Autodesk Inventor part; units mm, degrees
ref_plane "YZ Plane" through (0, 0, 0) normal (1, 0, 0) x (0, 1, 0)
ref_plane "XZ Plane" through (0, 0, 0) normal (0, 1, 0) x (-1, 0, 0)
ref_plane "XY Plane" through (0, 0, 0) normal (0, 0, 1) x (1, 0, 0)
sketch "스케치1" plane through (0, 0, 0) normal (0, 0, 1) x (1, 0, 0)
  line L0 (16.3992, -9.8355) -> (-16.3992, -9.8355)
  line L1 (-16.3992, -9.8355) -> (-16.3992, 9.8355)
  line L2 (-16.3992, 9.8355) -> (16.3992, 9.8355)
  line L3 (16.3992, 9.8355) -> (16.3992, -9.8355)
  line L4 (16.3992, -9.8355) -> (-16.3992, 9.8355) construction
  line L5 (-16.3992, -9.8355) -> (16.3992, 9.8355) construction
  point P0 (0, 0)
extrude "돌출1" add sketch "스케치1" along normal blind 15
sketch "스케치2" plane through (0, 0, 15) normal (0, 0, 1) x (1, 0, 0)
  line L0 (-16.3992, 9.8355) -> (-16.3992, -9.8355)
  line L1 (-16.3992, -9.8355) -> (16.3992, -9.8355)
  line L2 (-16.3992, -0.8122) -> (-1.2307, -0.8122)
  line L3 (-1.2307, -0.8122) -> (-1.2307, -9.8355)
  line L4 (-1.2307, -9.8355) -> (-16.3992, -9.8355)
  line L5 (-16.3992, -9.8355) -> (-16.3992, -0.8122)
  point P0 (0, 0)
extrude "돌출2" add sketch "스케치2" along normal blind 5
sketch "스케치3" plane through (0, 0, 15) normal (0, 0, 1) x (1, 0, 0)
  point P0 (0, 0)
sketch "스케치4" plane through (0, 0, 0) normal (0, 0, -1) x (-1, 0, 0)
  line L0 (-16.3992, 9.8355) -> (16.3992, 9.8355)
  circle A0 centre (0, 9.8355) radius 14.5299
  point P0 (0, 0)
extrude "돌출3" cut sketch "스케치4" against normal blind 20
fillet "모깎기1" radius 2 1 edges at (16.3992, -9.8355, 7.5)
fillet "모깎기2" radius 2 1 edges at (-16.3992, -9.8355, 10)
properties part number "240503_3Dsketch12"
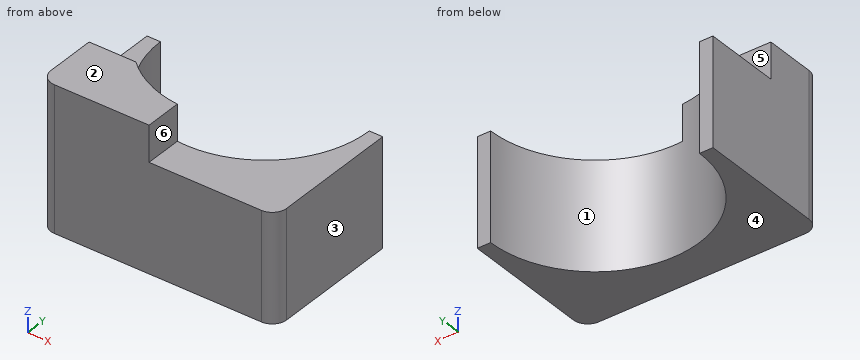
Geometry: final body of the model. Coordinates: model frame, mm. Face numbers are marked on the shaded views. A direction names the side the tool comes from. Round coordinates to 2 decimals unless told otherwise and drop trailing zeros. Loops run counter-clockwise (first coordinate to the right, second up) from the corner with the lowest first, then second, coordinate; pieces in that order, holes last. Notation, with made-up numbers: (-28, 60) -> (7, 60) arc R35 ccw to (7, 99) -> close; hole circle Ø7 at (89, 58.5). An arc over 180 degrees is marked (long way). Use one line per item in the form item = value. Start each with the question number.
1) Section D-D on y = 0.5. Output: boundary loops of the cut face in (x, z), then the cut area to 3 significant figures.
2) Section C-C on x = 4.5. Output: boundary loops of the cut face in (y, z).
3) Access query for the marked faces 4, 5 and 6. Directions: +Z, -Z, +X, -X, +Y, -Y. A direction counts if a zero-diameter tool reaches every point of the face in a straight line with its end or side. Return the directions, or none.
4) Section B-B on z = 3.5. Output: boundary loops of the cut face in (x, y), then the cut area to 3 significant figures.
5) Section A-A on y = 8.25. Output: boundary loops of the cut face in (x, z), then the cut area to 3 significant figures.
6) Draft query along X for the marked faces 1, 2 and 3. Return one class per face: released by +X, released by -X, zero draft, split by the parting line, or undercut.
7) First-contact query: P1, Ø5, axis at x = 6.5, z = 16.5, coming from the +Y side; P2, Ø5, axis at x = -12.5, y = 2.5, coming from the +Z side; P3, Ø6, axis at y = 3.5, z = 16, coming from the -X side; P4, Ø2.5, axis at y = -8.5, z = 17, coming from the +X side. Flat tips, straight axial feed; report the tip coordinate or a pass-through.
8) Line query: L1, parallel to X at y = -8, z = 10; L2, parallel to X at y = -5.25, z = 16.25; L3, parallel to Y at x = 0.5, z = 12.5. Output: solid intervals per line, ascending.
Response:
q1.outline = (-16.4, 0) -> (-11.13, 0) -> (-11.13, 15) -> (-16.4, 15) -> close; (11.13, 0) -> (16.4, 0) -> (16.4, 15) -> (11.13, 15) -> close
q1.area = 158 mm^2
q2.outline = (-9.84, 0) -> (-3.98, 0) -> (-3.98, 15) -> (-9.84, 15) -> close
q3.face_4 = -Z, +X, -X, +Y, -Y
q3.face_5 = +Z, +X, -X, +Y
q3.face_6 = +Z, +X, +Y, -Y
q4.outline = (-16.4, -7.84) arc R2 ccw to (-14.4, -9.84) -> (14.4, -9.84) arc R2 ccw to (16.4, -7.84) -> (16.4, 9.84) -> (14.53, 9.84) arc R14.53 cw to (-14.53, 9.84) -> (-16.4, 9.84) -> close
q4.area = 312 mm^2
q5.outline = (-16.4, 0) -> (-14.44, 0) -> (-14.44, 15) -> (-16.4, 15) -> close; (14.44, 0) -> (16.4, 0) -> (16.4, 15) -> (14.44, 15) -> close
q5.area = 58.7 mm^2
q6.face_1 = undercut
q6.face_2 = zero draft
q6.face_3 = released by +X
q7.P1 = -1.95
q7.P2 = 15
q7.P3 = -16.4
q7.P4 = -1.23
q8.L1 = -16.39 to 16.39
q8.L2 = -16.4 to -1.23
q8.L3 = -9.84 to -4.69
